Geometry check sheet. Reference: drawing and pictorial views, mm from the part's lowest x, y, z. A direction names the side the tool comes from. Give positions to 0.01 mm unless a question says otherwise; leave off trailing zeros. Order: outer loops, then holes, each group sorted by start corner. A loop starts at its lowest first (then second) coordinate and runs counter-clockwise, first axis right, second up.
Item 1: Sectioned sample at A-A on x = 31. Record the boundary of the cut face in (y, z), and give its area (3 significant figures).
Item 2: Gauge pin test, flat ends, axial feed: P1, Ø10, axis at x = 46, z = 6.5, coming from the +Y side; P2, Ø10, axis at x = 28, y = 46.5, coming from the +Z side. Record the tip position at first contact, or that the pin passes through.
Item 3: Sectioned sample at B-B on z = 31. Record the boundary of the cut face in (x, y), and give its area (3 significant figures).
Item 4: Material ranges on line 1 along Y through (x, z) = (32.5, 4); line 2 along Y through (x, z) = (33, 48); line 3 along X through (y, z) = (38, 34), recorded low to high.
Item 5: Sectioned sample at D-D on z = 12. Record the boundary of the cut face in (x, y).
Item 6: Sectioned sample at C-C on y = 33. Record the boundary of the cut face in (x, z).
Item 7: Access from +Z, -Z, +X, -X, +Y, -Y to the whole of each face (thin tool, end or side, straight path). Record for the marked faces 1 and 2.
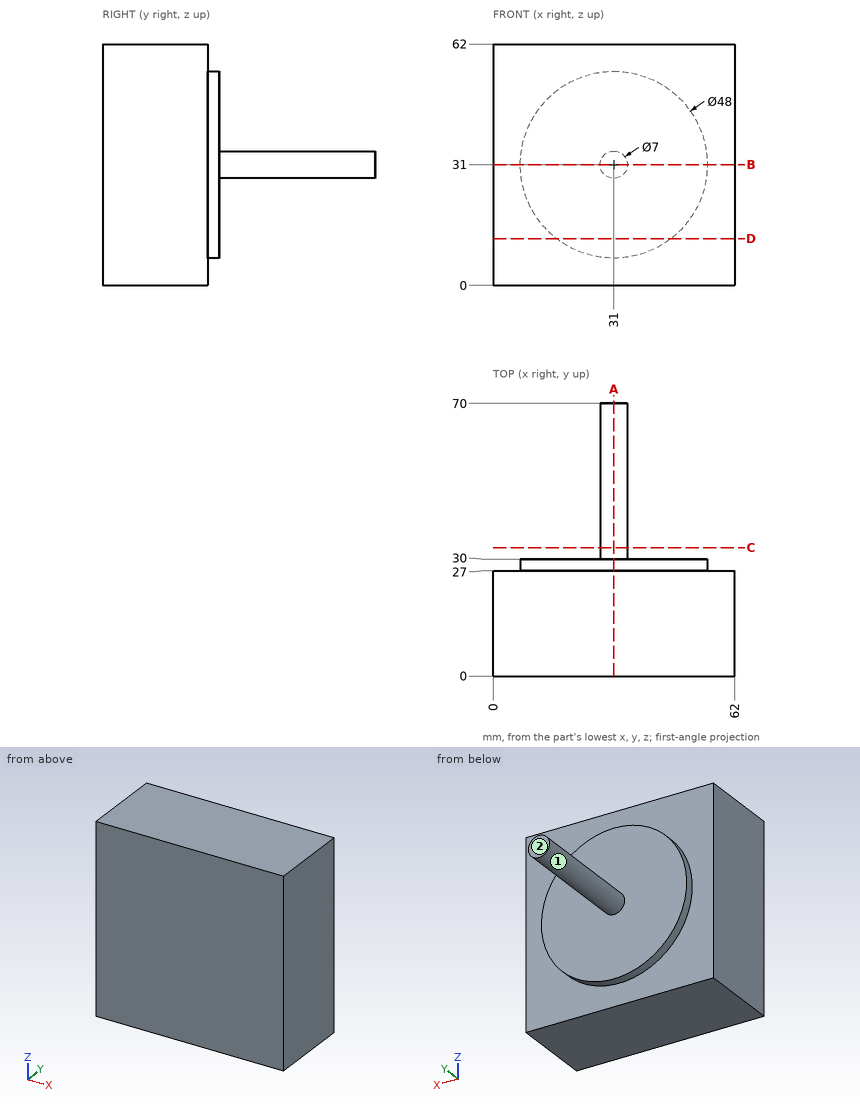
Report:
1. outline: (0, 0) - (27, 0) - (27, 7) - (30, 7) - (30, 27.5) - (70, 27.5) - (70, 34.5) - (30, 34.5) - (30, 55) - (27, 55) - (27, 62) - (0, 62) - close
1. area: 2,100 mm2
2. P1: stops at y = 30
2. P2: stops at z = 34.5
3. outline: (0, 0) - (62, 0) - (62, 27) - (55, 27) - (55, 30) - (34.5, 30) - (34.5, 70) - (27.5, 70) - (27.5, 30) - (7, 30) - (7, 27) - (0, 27) - close
3. area: 2,100 mm2
4. line 1: y = 0 to 27
4. line 2: y = 0 to 30
4. line 3: x = 29.2 to 32.8
5. outline: (0, 0) - (62, 0) - (62, 27) - (45.66, 27) - (45.66, 30) - (16.34, 30) - (16.34, 27) - (0, 27) - close
6. outline: circle Ø7 at (31, 31)
7. face 1: +Y
7. face 2: +Z, -Z, +X, -X, +Y
